```python
from build123d import *

# Parameters (mm, degrees)
SKETCH1_R           = 30
SKETCH1_R_2         = 5
SKETCH1_R_3         = 8
SKETCH1_R_4         = 1.5
SKETCH1_R_5         = 11
BOSS_EXTRUDE1_DEPTH = 3
CUT_EXTRUDE1_START  = -10
SKETCH2_R           = 8
SKETCH2_R_2         = 1.5
CUT_EXTRUDE1_DEPTH  = 10


with BuildPart() as part:
    # Sketch1 → Boss-Extrude1 (new body)
    with BuildSketch(Plane(origin=(0, 0, 0), x_dir=(1, 0, 0), z_dir=(0, 1, 0))):
        with BuildLine():
            Line((9.113159771, 23.279826438), (-27.083788873, 37.44954446))
            ThreePointArc((-27.083788873, 37.44954446), (-36.443445881, 34.74151929), (-36.244997998, 25))
            Line((-36.244997998, 25), (-22, -11.874342087))
            ThreePointArc((-22, -11.874342087), (-19.917132472, -15.109858837), (-17.362407178, -17.987407178))
            Line((-17.362407178, -17.987407178), (6.954011254, -41.458914425))
            ThreePointArc((6.954011254, -41.458914425), (11.530098852, -96.683349609), (66.881782611, -99.30440362))
            Line((66.881782611, -99.30440362), (186.110074258, -214.389925742))
            ThreePointArc((186.110074258, -214.389925742), (206.945082055, -214.389810698), (207.681250796, -193.567812582))
            Line((207.681250796, -193.567812582), (18.589553719, 16.716114756))
            ThreePointArc((18.589553719, 16.716114756), (14.234839706, 20.551626178), (9.113159771, 23.279826438))
        make_face()
        with Locations(Location((40.698942911, -66.46450555, 0), (0, 0, 270))):
            Circle(SKETCH1_R, mode=Mode.SUBTRACT)
        with Locations(Location((-30, 30, 0), (0, 0, 270))):
            Circle(SKETCH1_R_2, mode=Mode.SUBTRACT)
        with Locations(Location((0, 0, 0), (0, 0, 270))):
            Circle(SKETCH1_R_3, mode=Mode.SUBTRACT)
        with Locations(Location((57.698942911, -37.019641821, 0), (0, 0, 270))):
            Circle(SKETCH1_R_4, mode=Mode.SUBTRACT)
        with Locations(Location((23.698942911, -37.019641821, 0), (0, 0, 270))):
            Circle(SKETCH1_R_4, mode=Mode.SUBTRACT)
        with Locations(Location((74.698942911, -66.46450555, 0), (0, 0, 270))):
            Circle(SKETCH1_R_4, mode=Mode.SUBTRACT)
        with Locations(Location((6.698942911, -66.46450555, 0), (0, 0, 270))):
            Circle(SKETCH1_R_4, mode=Mode.SUBTRACT)
        with Locations(Location((57.698942911, -95.909369279, 0), (0, 0, 270))):
            Circle(SKETCH1_R_4, mode=Mode.SUBTRACT)
        with Locations(Location((23.698942911, -95.909369279, 0), (0, 0, 270))):
            Circle(SKETCH1_R_4, mode=Mode.SUBTRACT)
        with Locations(Location((196.527518564, -203.597481436, 0), (0, 0, 270))):
            Circle(SKETCH1_R_5, mode=Mode.SUBTRACT)
    extrude(amount=BOSS_EXTRUDE1_DEPTH)

    # Sketch2 → Cut-Extrude1 (cut)
    with BuildSketch(Plane(origin=(0, 3, 0), x_dir=(1, 0, 0), z_dir=(0, 1, 0)).offset(CUT_EXTRUDE1_START)):
        with Locations(Location((0, 0, 0), (0, 0, 270))):
            Circle(SKETCH2_R)
        with Locations(Location((-15.62616646, -16.18866646, 0), (0, 0, 270))):
            Circle(SKETCH2_R_2)
        with Locations(Location((-2.656534873, -28.707648342, 0), (0, 0, 270))):
            Circle(SKETCH2_R_2)
        with Locations(Location((127.883379131, -154.711753185, 0), (0, 0, 270))):
            Circle(SKETCH2_R_2)
        with Locations(Location((100.268681967, -128.056570951, 0), (0, 0, 270))):
            Circle(SKETCH2_R_2)
        with Locations(Location((155.700523111, -181.562347912, 0), (0, 0, 270))):
            Circle(SKETCH2_R_2)
        with Locations(Location((148.934969969, -131.976518297, 0), (0, 0, 270))):
            Circle(SKETCH2_R_2)
        with Locations(Location((177.993903369, -164.292197589, 0), (0, 0, 270))):
            Circle(SKETCH2_R_2)
        with Locations(Location((125.057017775, -105.422472605, 0), (0, 0, 270))):
            Circle(SKETCH2_R_2)
        with Locations(Location((49.600984197, -21.509792527, 0), (0, 0, 270))):
            Circle(SKETCH2_R_2)
        with Locations(Location((25.948559408, 4.79345004, 0), (0, 0, 270))):
            Circle(SKETCH2_R_2)
        with Locations(Location((-26.895954044, 7.736794096, 0), (0, 0, 270))):
            Circle(SKETCH2_R_2)
        with Locations(Location((-10.272154034, 28.183705865, 0), (0, 0, 270))):
            Circle(SKETCH2_R_2)
    extrude(amount=CUT_EXTRUDE1_DEPTH, mode=Mode.SUBTRACT)


solid = part.part
```
Model file for the job. Use its own axes, mm. A direction names the side the tool comes from. Coordinates: 2 decimals unless noted, no trailing zeros. Order: outer loops, then holes, each group sorted by start corner. A loop starts at its lowest first (then second) coordinate and runs counter-clockwise, first axis right, second up. Notation, with made-up numbers: (43.25, 79) -> (57.25, 79) arc R37 ccw to (57.25, 115) -> close; hole circle Ø11 at (67, 51.5). An arc over 180 degrees is marked (long way). Return JSON: item names as keys, results as strings.
Item 1: Slice it at B-B (y = 1.2). Count the separate pieces of the cut face and the enclosed holes in it, then the cut area to 3 significant figures.
Model answer:
{"separate pieces": "1", "enclosed holes": "22", "area": "12,000 mm²"}
Item 2: Wall check: line 1 along Z through (x, y) = (-2, 0.4); line 2 along Z through (x, y) = (4.5, 2.75); line 3 along Z through (x, y) = (33, 1.3). Give the ranges that are in metal, low to high. Write a range as from..to.
Model answer:
{"line 1": "z = -27.63..-7.75, 7.75..27.36, 30.06..32.82", "line 2": "z = -25.09..-6.61, 6.61..39.09, 45.17..87.76", "line 3": "z = -0.69..37.47, 95.46..107.75"}
Item 3: Slice it at D-D (x = 93). Write the cut outline in (y, z).
Model answer:
{"outline": "(0, 66.03) -> (3, 66.03) -> (3, 124.52) -> (0, 124.52) -> close"}
Item 4: Mould opens along X. For faces 1 (the face through (114.46, 1.48, 89.9)), 2 (the face through (-7.81, 1.48, -1.73)), 3 (the face through (206.71, 1.48, 214.61)) say: pulls with the +X half, pulls with the -X half, needs draft (parallel to the pull), parting line crosses it, or undercut.
Model answer:
{"face 1": "pulls with the +X half", "face 2": "undercut", "face 3": "parting line crosses it"}
Item 5: Slice it at C-C (z = 0). Write the cut outline in (x, y).
Model answer:
{"outline": "(-26.59, 0) -> (-8, 0) -> (-8, 3) -> (-26.59, 3) -> close; (8, 0) -> (33.62, 0) -> (33.62, 3) -> (8, 3) -> close"}
Item 6: Slice it at A-A (z = 47.5). Write the cut outline in (x, y).
Model answer:
{"outline": "(3.22, 0) -> (17.45, 0) -> (17.45, 3) -> (3.22, 3) -> close; (63.94, 0) -> (76.33, 0) -> (76.33, 3) -> (63.94, 3) -> close"}
Item 7: 3-axis set-ups, long thin cutter, end or side, ignore diameter. For faces 4 (the face through (-5.374, 1.479, 29.559)), 5 (the face through (14.302, 1.479, -20.505)): which of +Z, -Z, +X, -X, +Y, -Y reach the whole face in a straight line?
Model answer:
{"face 4": "-X, +Y, -Y", "face 5": "-Z, +X, +Y, -Y"}
Item 8: Pin check, flat tips, straight feed: P1, Ø1.5, axis at x = 179, y = 2, coming from the +Z side; P2, Ø1, axis at y = 1, z = 46, coming from the +X side; P3, Ø2.5, axis at x = 25.95, z = -4.79, coming from the +Y side; P4, Ø4, axis at x = 49.6, z = 21.51, coming from the -Y side. Stop position of each tip, or through.
Model answer:
{"P1": "stops at z = 208.25", "P2": "stops at x = 75.43", "P3": "passes through", "P4": "stops at y = 0"}
